```python
from build123d import *

# Parameters (mm, degrees)
SKETCH_1_W           = 93.98
SKETCH_1_H           = 63.5
SKETCH_1_R           = 1.05
EXTRUDE_1_DEPTH      = 4
SKETCH_2_OUTSIDE_W   = 118.678
SKETCH_2_OUTSIDE_H   = 88.198
SKETCH_2_OUTSIDE_W_2 = 5.08
SKETCH_2_OUTSIDE_H_2 = 5.08
CUT_EXTRUDE_1_DEPTH  = 1.5
SKETCH_3_R           = 2.6
CUT_EXTRUDE_2_DEPTH  = 0.8


with BuildPart() as part:
    # 草图1 → 凸台-拉伸1 (new body)
    with BuildSketch(Plane(origin=(0, 0, 0), x_dir=(1, 0, 0), z_dir=(0, 1, 0))):
        Rectangle(SKETCH_1_W, SKETCH_1_H)
        with Locations(Location((-44.45, 29.21, 0), (0, 0, 270))):
            Circle(SKETCH_1_R, mode=Mode.SUBTRACT)
        with Locations(Location((-44.45, -29.21, 0), (0, 0, 270))):
            Circle(SKETCH_1_R, mode=Mode.SUBTRACT)
        with Locations(Location((44.45, 29.21, 0), (0, 0, 270))):
            Circle(SKETCH_1_R, mode=Mode.SUBTRACT)
        with Locations(Location((44.45, -29.21, 0), (0, 0, 270))):
            Circle(SKETCH_1_R, mode=Mode.SUBTRACT)
    extrude(amount=EXTRUDE_1_DEPTH)

    # 草图2 outside → 切除-拉伸1 (cut)
    with BuildSketch(Plane(origin=(0, 4, 0), x_dir=(1, 0, 0), z_dir=(0, 1, 0))):
        Rectangle(SKETCH_2_OUTSIDE_W, SKETCH_2_OUTSIDE_H)
        with Locations((-44.45, 29.21)):
            Rectangle(SKETCH_2_OUTSIDE_W_2, SKETCH_2_OUTSIDE_H_2, mode=Mode.SUBTRACT)
        with Locations((-44.45, -29.21)):
            Rectangle(SKETCH_2_OUTSIDE_W_2, SKETCH_2_OUTSIDE_H_2, mode=Mode.SUBTRACT)
        with Locations((44.45, -29.21)):
            Rectangle(SKETCH_2_OUTSIDE_W_2, SKETCH_2_OUTSIDE_H_2, mode=Mode.SUBTRACT)
        with Locations((44.45, 29.21)):
            Rectangle(SKETCH_2_OUTSIDE_W_2, SKETCH_2_OUTSIDE_H_2, mode=Mode.SUBTRACT)
    extrude(amount=-CUT_EXTRUDE_1_DEPTH, mode=Mode.SUBTRACT)

    # 草图3 → 切除-拉伸2 (cut)
    with BuildSketch(Plane.XZ):
        with Locations(Location((-36.99, 21.75, 0), (0, 0, 270))):
            Circle(SKETCH_3_R)
        with Locations(Location((-36.99, -21.75, 0), (0, 0, 270))):
            Circle(SKETCH_3_R)
        with Locations(Location((0, 21.75, 0), (0, 0, 270))):
            Circle(SKETCH_3_R)
        with Locations(Location((0, -21.75, 0), (0, 0, 270))):
            Circle(SKETCH_3_R)
        with Locations(Location((36.99, 21.75, 0), (0, 0, 270))):
            Circle(SKETCH_3_R)
        with Locations(Location((36.99, -21.75, 0), (0, 0, 270))):
            Circle(SKETCH_3_R)
    extrude(amount=-CUT_EXTRUDE_2_DEPTH, mode=Mode.SUBTRACT)


solid = part.part
```
For this review, take the finished solid that the model builds, in its own axes (mm). A direction names the side the tool comes from. Round coordinates to 2 decimals unless told otherwise and drop trailing zeros. Write each loop counter-clockwise with the first axis right and the second up, starting at its lowest first coordinate (ties: lowest second). Pieces come first, ordered by that corner, then holes. Notation, with made-up numbers: (64, 23.5) - (109, 23.5) arc R27 ccw to (109, 40.5) - close; hole circle Ø2 at (81, -34). An arc over 180 degrees is marked (long way). Put each result on its own line as item: value.
Q1. Machinability: for faces 3 (the face through (43.81, 1.97, 28.38)), 4 (the face through (-34.412, 0.394, 22.088)), which of the approach directions +Z, -Z, +X, -X, +Y, -Y give a long, thin tool a straight path to every point of the face, cutting with its end or side? Answer none if there is none.
Solved:
face 3: +Y, -Y
face 4: -Y
Q2. We need section D-D (z = 14). Give the boundary of the cut face in (x, y).
Solved:
outline: (-46.99, 0) - (46.99, 0) - (46.99, 2.5) - (-46.99, 2.5) - close
Q3. We need section B-B (z = 21.75). Give the boundary of the cut face in (x, y).
Solved:
outline: (-46.99, 0) - (-39.59, 0) - (-39.59, 0.8) - (-34.39, 0.8) - (-34.39, 0) - (-2.6, 0) - (-2.6, 0.8) - (2.6, 0.8) - (2.6, 0) - (34.39, 0) - (34.39, 0.8) - (39.59, 0.8) - (39.59, 0) - (46.99, 0) - (46.99, 2.5) - (-46.99, 2.5) - close
Q4. Mouldability with a two-part tool opening along X and no side actions: class faces 1 (the face through (43, 4, -29)), 2 (the face through (0.78, 0.39, 19.27)) as released by +X, released by -X, zero draft, split by the parting line, or undercut.
Solved:
face 1: zero draft
face 2: undercut
Q5. We need section C-C (x = -23). Give the boundary of the cut face in (y, z), and give its area (3 significant figures).
Solved:
outline: (0, -31.75) - (2.5, -31.75) - (2.5, 31.75) - (0, 31.75) - close
area: 159 mm2
Q6. Wall thickness on probe 1 along X at (y, z) = (0.35, 21.75); probe 2 along X at (y, z) = (3.1, -29); probe 3 along X at (y, z) = (1, 29.21): over which ranges is each line inside the solid? List them lowest first.
Solved:
probe 1: x = -46.99 to -39.59, -34.39 to -2.6, 2.6 to 34.39, 39.59 to 46.99
probe 2: x = -46.99 to -45.48, -43.42 to -41.91, 41.91 to 43.42, 45.48 to 46.99
probe 3: x = -46.99 to -45.5, -43.4 to 43.4, 45.5 to 46.99
Q7. Insertion check: pin 1 Ø1.6 at (x, z) = (36.5, -22) entering from -Y; pin 2 Ø8.5 at (x, z) = (0, -21.75) entering from +Y. Each pin has a flat end and moves straight along its axis. Give the tip position at first contact, or say it passes through.
Solved:
pin 1: stops at y = 0.8
pin 2: stops at y = 2.5
Q8. We need section A-A (x = 44.45). Give the boundary of the cut face in (y, z).
Solved:
outline: (0, -31.75) - (4, -31.75) - (4, -30.26) - (0, -30.26) - close; (0, -28.16) - (4, -28.16) - (4, -26.67) - (2.5, -26.67) - (2.5, 26.67) - (4, 26.67) - (4, 28.16) - (0, 28.16) - close; (0, 30.26) - (4, 30.26) - (4, 31.75) - (0, 31.75) - close
